The figure shows three views and two pictorial views of one solid part (mm, origin at its lowest corner). Answer the questions. Coordinates: 2 decimals unless noted, no trailing zeros. Order: outer loops, then holes, each group sorted by start corner. A loop starts at its lowest first (then second) coordinate and runs counter-clockwise, first axis right, second up. Notation, with made-up numbers: (-25, -18) -> (-20, -18) arc R9 ccw to (-20, -13) -> close; hole circle Ø7 at (69.25, 89). An arc over 180 degrees is marked (long way). Use one line per item in the form item = value.
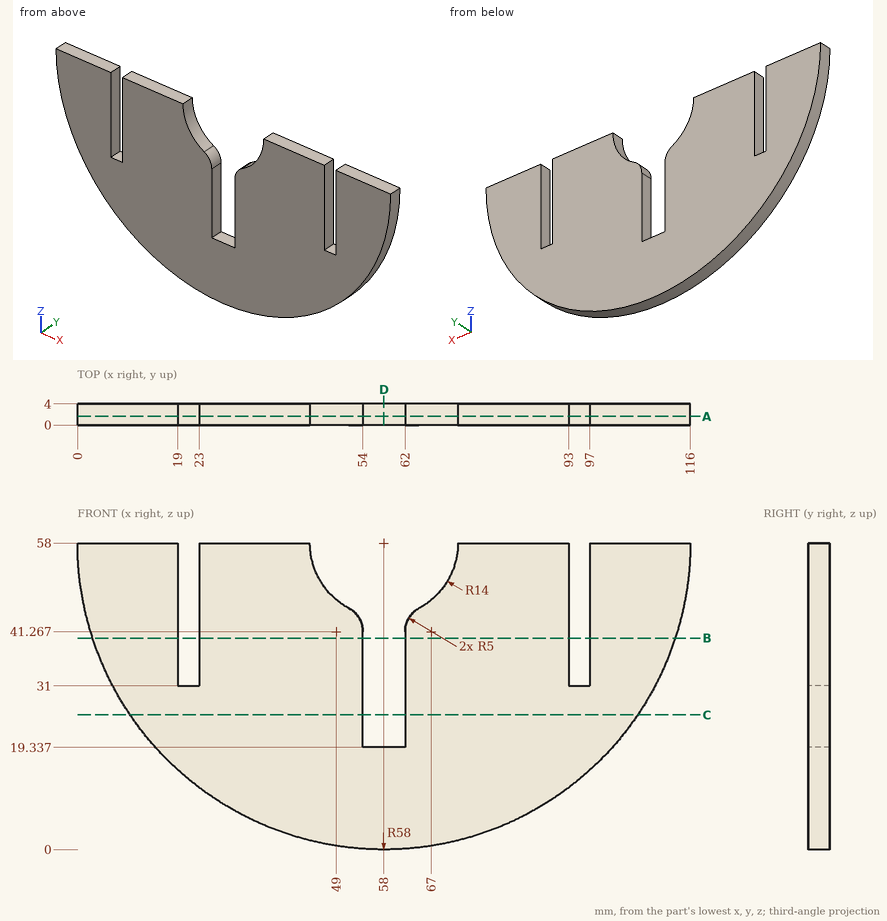
(1) Straight lines are drawn through the part: line 1 along X through (y, z) = (1.8, 51.5) (1 decimal); line 2 along X through (y, z) = (2.15, 39.5); line 3 along Z through (x, y) = (9.5, 1). For each, find the intervals that lie inside material, in ascending order.
Data:
line_1 = 0.4 to 19, 23 to 45.6, 70.4 to 93, 97 to 115.6
line_2 = 3.03 to 19, 23 to 54, 62 to 93, 97 to 112.97
line_3 = 26.19 to 58
(2) Section D-D on x = 58 is taken. Write down the section's boundary in (y, z).
Data:
outline = (0, 0) -> (4, 0) -> (4, 19.34) -> (0, 19.34) -> close
(3) Section B-B on z = 40 is taken. Write down the section's boundary in (x, y), plus the area to 3 significant figures.
Data:
outline = (2.86, 0) -> (19, 0) -> (19, 4) -> (2.86, 4) -> close; (23, 0) -> (54, 0) -> (54, 4) -> (23, 4) -> close; (62, 0) -> (93, 0) -> (93, 4) -> (62, 4) -> close; (97, 0) -> (113.14, 0) -> (113.14, 4) -> (97, 4) -> close
area = 377 mm²
(4) Section C-C on z = 25.5 is taken. Write down the section's boundary in (x, y).
Data:
outline = (9.96, 0) -> (54, 0) -> (54, 4) -> (9.96, 4) -> close; (62, 0) -> (106.04, 0) -> (106.04, 4) -> (62, 4) -> close
(5) Section A-A on y = 1.65 is taken. Write down the section's boundary in (x, z).
Data:
outline = (0, 58) arc R58 ccw to (116, 58) -> (97, 58) -> (97, 31) -> (93, 31) -> (93, 58) -> (72, 58) arc R14 cw to (64.63, 45.67) arc R5 ccw to (62, 41.27) -> (62, 19.34) -> (54, 19.34) -> (54, 41.27) arc R5 ccw to (51.37, 45.67) arc R14 cw to (44, 58) -> (23, 58) -> (23, 31) -> (19, 31) -> (19, 58) -> close
(6) Each of these flat-tipped pins is pushed along its axis until it touches: P1, Ø1.2, axis at x = 95.5, y = 2.5, coming from the +Z side; P2, Ø2, axis at y = 2, z = 30, coming from the +X side; P3, Ø1.2, axis at y = 1.5, z = 48.5, coming from the -X side. Where does it stop, or does it pass through?
Data:
P1 = 31
P2 = 109.33
P3 = 0.69
